Part model, mm, in its own coordinate system. Face numbers are marked on the shaded views. A direction names the side the tool comes from. Coordinates: 2 decimals unless noted, no trailing zeros. Write each loop counter-clockwise with the first axis right and the second up, starting at its lowest first coordinate (ties: lowest second). Pieces come first, ordered by that corner, then holes. Notation, with made-up numbers: (30, -6) - (82, -6) arc R30 ccw to (82, 26) - close; hole circle Ø7 at (66, 72). An arc over 180 degrees is marked (long way). Use a Markdown table: item, result.
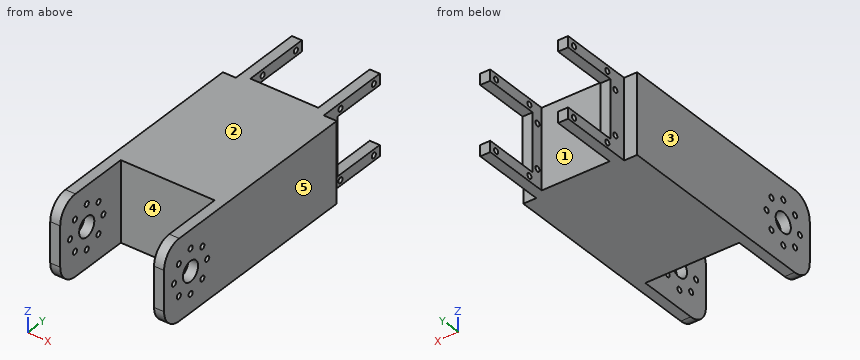
```python
from build123d import *

# Parameters (mm, degrees)
SKETCH2_W           = 34
SKETCH2_H           = 40
BOSS_EXTRUDE1_DEPTH = 3
SKETCH3_W           = 5
SKETCH3_H           = 40
BOSS_EXTRUDE2_DEPTH = 37
CUT_EXTRUDE1_REACH  = 72.036
SKETCH4_R           = 1.35
SKETCH4_W           = 29
SKETCH4_H           = 28
SKETCH5_W           = 57
SKETCH5_H           = 40
BOSS_EXTRUDE3_DEPTH = 3
SKETCH6_W           = 57
SKETCH6_H           = 40
SKETCH6_W_2         = 51
SKETCH6_H_2         = 34
BOSS_EXTRUDE4_DEPTH = 68.03
SKETCH7_W           = 57
SKETCH7_H           = 40
BOSS_EXTRUDE5_DEPTH = 3
SKETCH8_W           = 5
SKETCH8_H           = 40
BOSS_EXTRUDE6_DEPTH = 40
CUT_EXTRUDE2_REACH  = 135.611
SKETCH9_R           = 5
SKETCH9_R_2         = 1.35


with BuildPart() as part:
    # Sketch2 → Boss-Extrude1 (new body)
    with BuildSketch(Plane(origin=(0, 0, 0), x_dir=(1, 0, 0), z_dir=(0, 1, 0))):
        with Locations((17, 20)):
            Rectangle(SKETCH2_W, SKETCH2_H)
    extrude(amount=BOSS_EXTRUDE1_DEPTH)

    # Sketch3 → Boss-Extrude2 (add)
    with BuildSketch(Plane(origin=(0, 0, 0), x_dir=(1, 0, 0), z_dir=(0, 1, 0))):
        with Locations((-2.5, 20)):
            Rectangle(SKETCH3_W, SKETCH3_H)
        with Locations((36.5, 20)):
            Rectangle(SKETCH3_W, SKETCH3_H)
    extrude(amount=BOSS_EXTRUDE2_DEPTH)

    # Cut-Extrude1: up to this face of the body (flat: up to its plane)
    cut_extrude1_end = Plane(part.part.faces().sort_by_distance((39, 18.5, -20))[0])
    # Sketch4 → Cut-Extrude1 (cut, up to the picked face)
    with BuildSketch(Plane.ZY.offset(5), mode=Mode.PRIVATE) as cut_extrude1_sk1:
        with Locations((-2.8, 33.1)):
            Circle(SKETCH4_R)
    cut_extrude1_tool1 = split(extrude(cut_extrude1_sk1.sketch, amount=-CUT_EXTRUDE1_REACH, mode=Mode.PRIVATE), bisect_by=cut_extrude1_end, keep=Keep.BOTH, mode=Mode.PRIVATE)
    # Sketch4 → Cut-Extrude1 (cut, up to the picked face)
    with BuildSketch(Plane.ZY.offset(5), mode=Mode.PRIVATE) as cut_extrude1_sk2:
        with Locations((-2.8, 11.1)):
            Circle(SKETCH4_R)
    cut_extrude1_tool2 = split(extrude(cut_extrude1_sk2.sketch, amount=-CUT_EXTRUDE1_REACH, mode=Mode.PRIVATE), bisect_by=cut_extrude1_end, keep=Keep.BOTH, mode=Mode.PRIVATE)
    # Sketch4 → Cut-Extrude1 (cut, up to the picked face)
    with BuildSketch(Plane.ZY.offset(5), mode=Mode.PRIVATE) as cut_extrude1_sk3:
        with Locations((-9.1, 5.8)):
            Circle(SKETCH4_R)
    cut_extrude1_tool3 = split(extrude(cut_extrude1_sk3.sketch, amount=-CUT_EXTRUDE1_REACH, mode=Mode.PRIVATE), bisect_by=cut_extrude1_end, keep=Keep.BOTH, mode=Mode.PRIVATE)
    # Sketch4 → Cut-Extrude1 (cut, up to the picked face)
    with BuildSketch(Plane.ZY.offset(5), mode=Mode.PRIVATE) as cut_extrude1_sk4:
        with Locations((-37.4, 11.1)):
            Circle(SKETCH4_R)
    cut_extrude1_tool4 = split(extrude(cut_extrude1_sk4.sketch, amount=-CUT_EXTRUDE1_REACH, mode=Mode.PRIVATE), bisect_by=cut_extrude1_end, keep=Keep.BOTH, mode=Mode.PRIVATE)
    # Sketch4 → Cut-Extrude1 (cut, up to the picked face)
    with BuildSketch(Plane.ZY.offset(5), mode=Mode.PRIVATE) as cut_extrude1_sk5:
        with Locations((-31.1, 5.8)):
            Circle(SKETCH4_R)
    cut_extrude1_tool5 = split(extrude(cut_extrude1_sk5.sketch, amount=-CUT_EXTRUDE1_REACH, mode=Mode.PRIVATE), bisect_by=cut_extrude1_end, keep=Keep.BOTH, mode=Mode.PRIVATE)
    # Sketch4 → Cut-Extrude1 (cut, up to the picked face)
    with BuildSketch(Plane.ZY.offset(5), mode=Mode.PRIVATE) as cut_extrude1_sk6:
        with Locations((-37.4, 33.1)):
            Circle(SKETCH4_R)
    cut_extrude1_tool6 = split(extrude(cut_extrude1_sk6.sketch, amount=-CUT_EXTRUDE1_REACH, mode=Mode.PRIVATE), bisect_by=cut_extrude1_end, keep=Keep.BOTH, mode=Mode.PRIVATE)
    # Sketch4 → Cut-Extrude1 (cut, up to the picked face)
    with BuildSketch(Plane.ZY.offset(5), mode=Mode.PRIVATE) as cut_extrude1_sk7:
        with Locations((-20, 23)):
            Rectangle(SKETCH4_W, SKETCH4_H)
    cut_extrude1_tool7 = split(extrude(cut_extrude1_sk7.sketch, amount=-CUT_EXTRUDE1_REACH, mode=Mode.PRIVATE), bisect_by=cut_extrude1_end, keep=Keep.BOTH, mode=Mode.PRIVATE)
    add(cut_extrude1_tool1.solids().sort_by(Axis((-5, 33.1, -2.8), (1, 0, 0)))[0], mode=Mode.SUBTRACT)
    add(cut_extrude1_tool2.solids().sort_by(Axis((-5, 11.1, -2.8), (1, 0, 0)))[0], mode=Mode.SUBTRACT)
    add(cut_extrude1_tool3.solids().sort_by(Axis((-5, 5.8, -9.1), (1, 0, 0)))[0], mode=Mode.SUBTRACT)
    add(cut_extrude1_tool4.solids().sort_by(Axis((-5, 11.1, -37.4), (1, 0, 0)))[0], mode=Mode.SUBTRACT)
    add(cut_extrude1_tool5.solids().sort_by(Axis((-5, 5.8, -31.1), (1, 0, 0)))[0], mode=Mode.SUBTRACT)
    add(cut_extrude1_tool6.solids().sort_by(Axis((-5, 33.1, -37.4), (1, 0, 0)))[0], mode=Mode.SUBTRACT)
    add(cut_extrude1_tool7.solids().sort_by(Axis((-5, 23, -20), (1, 0, 0)))[0], mode=Mode.SUBTRACT)

    # Sketch5 → Boss-Extrude3 (add)
    with BuildSketch(Plane(origin=(0, 0, 0), x_dir=(-1, 0, 0), z_dir=(0, -1, 0))):
        with Locations((-17, 20)):
            Rectangle(SKETCH5_W, SKETCH5_H)
    extrude(amount=BOSS_EXTRUDE3_DEPTH)

    # Sketch6 → Boss-Extrude4 (add)
    with BuildSketch(Plane.XZ.offset(3)):
        with Locations((17, -20)):
            Rectangle(SKETCH6_W, SKETCH6_H)
        with Locations((17, -20)):
            Rectangle(SKETCH6_W_2, SKETCH6_H_2, mode=Mode.SUBTRACT)
    extrude(amount=BOSS_EXTRUDE4_DEPTH)

    # Sketch7 → Boss-Extrude5 (add)
    with BuildSketch(Plane.XZ.offset(71.03)):
        with Locations((17, -20)):
            Rectangle(SKETCH7_W, SKETCH7_H)
    extrude(amount=BOSS_EXTRUDE5_DEPTH)

    # Sketch8 → Boss-Extrude6 (add)
    with BuildSketch(Plane.XZ.offset(74.03)):
        with Locations((-9, -20)):
            Rectangle(SKETCH8_W, SKETCH8_H)
        with Locations((43, -20)):
            Rectangle(SKETCH8_W, SKETCH8_H)
    extrude(amount=BOSS_EXTRUDE6_DEPTH)

    # Cut-Extrude2: up to this face of the body (flat: up to its plane)
    cut_extrude2_end = Plane(part.part.faces().sort_by_distance((-11.5, -57.015, -20))[0])
    # Sketch9 → Cut-Extrude2 (cut, up to the picked face)
    with BuildSketch(Plane(origin=(45.5, 0, 0), x_dir=(0, 0, -1), z_dir=(1, 0, 0)), mode=Mode.PRIVATE) as cut_extrude2_sk1:
        with BuildLine():
            ThreePointArc((40, -104.03), (37.071067812, -111.101067812), (30, -114.03))
            Line((30, -114.03), (40, -114.03))
            Line((40, -114.03), (40, -104.03))
        make_face()
    cut_extrude2_tool1 = split(extrude(cut_extrude2_sk1.sketch, amount=-CUT_EXTRUDE2_REACH, mode=Mode.PRIVATE), bisect_by=cut_extrude2_end, keep=Keep.BOTH, mode=Mode.PRIVATE)
    # Sketch9 → Cut-Extrude2 (cut, up to the picked face)
    with BuildSketch(Plane(origin=(45.5, 0, 0), x_dir=(0, 0, -1), z_dir=(1, 0, 0)), mode=Mode.PRIVATE) as cut_extrude2_sk2:
        with BuildLine():
            ThreePointArc((10, -114.03), (2.928932188, -111.101067812), (0, -104.03))
            Line((0, -104.03), (0, -114.03))
            Line((0, -114.03), (10, -114.03))
        make_face()
    cut_extrude2_tool2 = split(extrude(cut_extrude2_sk2.sketch, amount=-CUT_EXTRUDE2_REACH, mode=Mode.PRIVATE), bisect_by=cut_extrude2_end, keep=Keep.BOTH, mode=Mode.PRIVATE)
    # Sketch9 → Cut-Extrude2 (cut, up to the picked face)
    with BuildSketch(Plane(origin=(45.5, 0, 0), x_dir=(0, 0, -1), z_dir=(1, 0, 0)), mode=Mode.PRIVATE) as cut_extrude2_sk3:
        with Locations((20, -96.53)):
            Circle(SKETCH9_R)
    cut_extrude2_tool3 = split(extrude(cut_extrude2_sk3.sketch, amount=-CUT_EXTRUDE2_REACH, mode=Mode.PRIVATE), bisect_by=cut_extrude2_end, keep=Keep.BOTH, mode=Mode.PRIVATE)
    # Sketch9 → Cut-Extrude2 (cut, up to the picked face)
    with BuildSketch(Plane(origin=(45.5, 0, 0), x_dir=(0, 0, -1), z_dir=(1, 0, 0)), mode=Mode.PRIVATE) as cut_extrude2_sk4:
        with Locations((27.778174593, -104.308174593)):
            Circle(SKETCH9_R_2)
    cut_extrude2_tool4 = split(extrude(cut_extrude2_sk4.sketch, amount=-CUT_EXTRUDE2_REACH, mode=Mode.PRIVATE), bisect_by=cut_extrude2_end, keep=Keep.BOTH, mode=Mode.PRIVATE)
    # Sketch9 → Cut-Extrude2 (cut, up to the picked face)
    with BuildSketch(Plane(origin=(45.5, 0, 0), x_dir=(0, 0, -1), z_dir=(1, 0, 0)), mode=Mode.PRIVATE) as cut_extrude2_sk5:
        with Locations((20, -107.53)):
            Circle(SKETCH9_R_2)
    cut_extrude2_tool5 = split(extrude(cut_extrude2_sk5.sketch, amount=-CUT_EXTRUDE2_REACH, mode=Mode.PRIVATE), bisect_by=cut_extrude2_end, keep=Keep.BOTH, mode=Mode.PRIVATE)
    # Sketch9 → Cut-Extrude2 (cut, up to the picked face)
    with BuildSketch(Plane(origin=(45.5, 0, 0), x_dir=(0, 0, -1), z_dir=(1, 0, 0)), mode=Mode.PRIVATE) as cut_extrude2_sk6:
        with Locations((12.221825407, -104.308174593)):
            Circle(SKETCH9_R_2)
    cut_extrude2_tool6 = split(extrude(cut_extrude2_sk6.sketch, amount=-CUT_EXTRUDE2_REACH, mode=Mode.PRIVATE), bisect_by=cut_extrude2_end, keep=Keep.BOTH, mode=Mode.PRIVATE)
    # Sketch9 → Cut-Extrude2 (cut, up to the picked face)
    with BuildSketch(Plane(origin=(45.5, 0, 0), x_dir=(0, 0, -1), z_dir=(1, 0, 0)), mode=Mode.PRIVATE) as cut_extrude2_sk7:
        with Locations((31, -96.53)):
            Circle(SKETCH9_R_2)
    cut_extrude2_tool7 = split(extrude(cut_extrude2_sk7.sketch, amount=-CUT_EXTRUDE2_REACH, mode=Mode.PRIVATE), bisect_by=cut_extrude2_end, keep=Keep.BOTH, mode=Mode.PRIVATE)
    # Sketch9 → Cut-Extrude2 (cut, up to the picked face)
    with BuildSketch(Plane(origin=(45.5, 0, 0), x_dir=(0, 0, -1), z_dir=(1, 0, 0)), mode=Mode.PRIVATE) as cut_extrude2_sk8:
        with Locations((27.778174593, -88.751825407)):
            Circle(SKETCH9_R_2)
    cut_extrude2_tool8 = split(extrude(cut_extrude2_sk8.sketch, amount=-CUT_EXTRUDE2_REACH, mode=Mode.PRIVATE), bisect_by=cut_extrude2_end, keep=Keep.BOTH, mode=Mode.PRIVATE)
    # Sketch9 → Cut-Extrude2 (cut, up to the picked face)
    with BuildSketch(Plane(origin=(45.5, 0, 0), x_dir=(0, 0, -1), z_dir=(1, 0, 0)), mode=Mode.PRIVATE) as cut_extrude2_sk9:
        with Locations((20, -85.53)):
            Circle(SKETCH9_R_2)
    cut_extrude2_tool9 = split(extrude(cut_extrude2_sk9.sketch, amount=-CUT_EXTRUDE2_REACH, mode=Mode.PRIVATE), bisect_by=cut_extrude2_end, keep=Keep.BOTH, mode=Mode.PRIVATE)
    # Sketch9 → Cut-Extrude2 (cut, up to the picked face)
    with BuildSketch(Plane(origin=(45.5, 0, 0), x_dir=(0, 0, -1), z_dir=(1, 0, 0)), mode=Mode.PRIVATE) as cut_extrude2_sk10:
        with Locations((12.221825407, -88.751825407)):
            Circle(SKETCH9_R_2)
    cut_extrude2_tool10 = split(extrude(cut_extrude2_sk10.sketch, amount=-CUT_EXTRUDE2_REACH, mode=Mode.PRIVATE), bisect_by=cut_extrude2_end, keep=Keep.BOTH, mode=Mode.PRIVATE)
    # Sketch9 → Cut-Extrude2 (cut, up to the picked face)
    with BuildSketch(Plane(origin=(45.5, 0, 0), x_dir=(0, 0, -1), z_dir=(1, 0, 0)), mode=Mode.PRIVATE) as cut_extrude2_sk11:
        with Locations((9, -96.53)):
            Circle(SKETCH9_R_2)
    cut_extrude2_tool11 = split(extrude(cut_extrude2_sk11.sketch, amount=-CUT_EXTRUDE2_REACH, mode=Mode.PRIVATE), bisect_by=cut_extrude2_end, keep=Keep.BOTH, mode=Mode.PRIVATE)
    add(cut_extrude2_tool1.solids().sort_by(Axis((45.5, -111.796321, -37.766321), (-1, 0, 0)))[0], mode=Mode.SUBTRACT)
    add(cut_extrude2_tool2.solids().sort_by(Axis((45.5, -111.796321, -2.233679), (-1, 0, 0)))[0], mode=Mode.SUBTRACT)
    add(cut_extrude2_tool3.solids().sort_by(Axis((45.5, -96.53, -20), (-1, 0, 0)))[0], mode=Mode.SUBTRACT)
    add(cut_extrude2_tool4.solids().sort_by(Axis((45.5, -104.308175, -27.778175), (-1, 0, 0)))[0], mode=Mode.SUBTRACT)
    add(cut_extrude2_tool5.solids().sort_by(Axis((45.5, -107.53, -20), (-1, 0, 0)))[0], mode=Mode.SUBTRACT)
    add(cut_extrude2_tool6.solids().sort_by(Axis((45.5, -104.308175, -12.221825), (-1, 0, 0)))[0], mode=Mode.SUBTRACT)
    add(cut_extrude2_tool7.solids().sort_by(Axis((45.5, -96.53, -31), (-1, 0, 0)))[0], mode=Mode.SUBTRACT)
    add(cut_extrude2_tool8.solids().sort_by(Axis((45.5, -88.751825, -27.778175), (-1, 0, 0)))[0], mode=Mode.SUBTRACT)
    add(cut_extrude2_tool9.solids().sort_by(Axis((45.5, -85.53, -20), (-1, 0, 0)))[0], mode=Mode.SUBTRACT)
    add(cut_extrude2_tool10.solids().sort_by(Axis((45.5, -88.751825, -12.221825), (-1, 0, 0)))[0], mode=Mode.SUBTRACT)
    add(cut_extrude2_tool11.solids().sort_by(Axis((45.5, -96.53, -9), (-1, 0, 0)))[0], mode=Mode.SUBTRACT)


solid = part.part
```
Item 1: Which spindle directions (+Z, -Z, +X, -X, +Y, -Y) get a long thin tool onto all of the face, cutting with end or side? Do the marked faces 4 and 5. Say none if no direction does.
From the geometry:
| item | result |
|---|---|
| face 4 | +Z, -Z, -Y |
| face 5 | +Z, -Z, +X, +Y, -Y |
Item 2: Band-saw the part on A-A, the plane y = 33.1. Count the separate pieces of the cut face and the enclosed holes in it, then the cut area to 3 significant figures.
From the geometry:
| item | result |
|---|---|
| separate pieces | 8 |
| enclosed holes | 0 |
| area | 56.0 mm^2 |
Item 3: Band-saw the part on C-C, the plane x = 5.5. Give the cut face in (y, z).
From the geometry:
| item | result |
|---|---|
| outline | (-74.03, -40) - (3, -40) - (3, 0) - (-74.03, 0) - close; hole (-71.03, -37) - (-3, -37) - (-3, -3) - (-71.03, -3) - close |
Item 4: Drop flat-ended pins along their axis: P1, Ø1.6, axis at y = -104.31, z = -12.22, coming from the -X side; P2, Ø3, axis at x = -7.5, z = -19.5, coming from the +Y side; P3, Ø10, axis at x = 11, z = -17.5, coming from the -Y side; P4, Ø17, axis at y = 20.5, z = -29, coming from the +X side. Give the stop position or say it passes through.
From the geometry:
| item | result |
|---|---|
| P1 | through |
| P2 | y = 0 |
| P3 | y = -74.03 |
| P4 | x = 39 |
Item 5: Drill centre lines: probe 1 along Y at (x, z) = (-2.65, -2.8); probe 2 along X at (y, z) = (-44, -35.5); probe 3 along X at (y, z) = (-75.5, -5.5). Where is each one in solid material? Low to high.
From the geometry:
| item | result |
|---|---|
| probe 1 | -74.03 to 9.75, 12.45 to 31.75, 34.45 to 37 |
| probe 2 | -11.5 to -8.5, 42.5 to 45.5 |
| probe 3 | -11.5 to -6.5, 40.5 to 45.5 |
Item 6: Band-saw the part on D-D, the plane y = 5.8. Give the cut face in (x, z).
From the geometry:
| item | result |
|---|---|
| outline | (-5, -40) - (0, -40) - (0, -32.45) - (-5, -32.45) - close; (-5, -29.75) - (0, -29.75) - (0, -10.45) - (-5, -10.45) - close; (-5, -7.75) - (0, -7.75) - (0, 0) - (-5, 0) - close; (34, -40) - (39, -40) - (39, -32.45) - (34, -32.45) - close; (34, -29.75) - (39, -29.75) - (39, -10.45) - (34, -10.45) - close; (34, -7.75) - (39, -7.75) - (39, 0) - (34, 0) - close |
Item 7: Two-plate mould, pull along X, no slides. Class the marked faces 1, 2 and 3: pulls with the +X half, pulls with the -X half, needs draft (parallel to the pull), parting line crosses it, or undercut.
From the geometry:
| item | result |
|---|---|
| face 1 | undercut |
| face 2 | needs draft |
| face 3 | pulls with the -X half |
